For this review, take the finished solid that the model builds, in its own axes (mm). Face numbers are marked on the shaded views. A direction names the side the tool comes from. Coordinates: 2 decimals unless noted, no trailing zeros. Loops run counter-clockwise (first coordinate to the right, second up) from the corner with the lowest first, then second, coordinate; pieces in that order, holes last. Notation, with made-up numbers: (-9.75, 36) - (13.25, 36) arc R24 ccw to (13.25, 60) - close; hole circle Ø4 at (72, -11). An arc over 180 degrees is marked (long way). One line per item, written item: value. Start each with the question number.
1. Take a section at C-C, the plane z = 5.5. State the section outline as (x, y) points, and give its area (3 significant figures).
2. For the marked faces 5, 6 and 7, list the 3-axis set-ups (+Z, -Z, +X, -X, +Y, -Y) from which the entire face can be reached by the end or side of a thin tool; tool diameter is ignored.
3. The part is to be moulded in two halves that separate along X. For the marked faces 1, 2, 3 and 4, say which applies: released by +X, released by -X, zero draft, split by the parting line, or undercut.
4. Insertion check: pin 1 (7.5 mm diameter, centred on x = 22.01, y = 142.89, fed in from -Z); pin 2 (1.8 mm diameter, centred on x = 22.5, y = 144, fed in from +Z). Each pin has a flat end and moves straight along its axis. Give the tip position at first contact, or say it passes through.
5. Take a section at B-B, the plane x = 15. State the section outline as (y, z) points.
6. To check wall thickness, follow line 1 (X direction, y = 162.5, z = 3.75); line 2 (Z direction, x = 9, y = 157); line 3 (X direction, y = 158.5, z = 0.75). State the ranges of each line that lie inside material, in increasing order. Write a range as from..to.
Autodesk Inventor part; units mm, degrees
ref_plane "YZ Plane" through (0, 0, 0) normal (1, 0, 0) x (0, 1, 0)
ref_plane "XZ Plane" through (0, 0, 0) normal (0, 1, 0) x (-1, 0, 0)
ref_plane "XY Plane" through (0, 0, 0) normal (0, 0, 1) x (1, 0, 0)
ref_plane "Work Plane1" through (52.5141, 202.7033, 6.4479) normal (0, 0, -1) x (0, 1, 0)
sketch "Sketch1" plane through (52.5141, 202.7033, 6.4479) normal (0, 0, -1) x (0, 1, 0)
  circle A0 centre (-59.8114, -30.5) radius 1.4 construction
  circle A1 centre (-38.8114, -18.3756) radius 1.4
  circle A2 centre (-38.8114, -42.6244) radius 1.4 construction
  circle A3 centre (41, 0) radius 1.65
  circle A4 centre (-9, 0) radius 1.65
  circle A5 centre (-9, 50) radius 1.65
  circle A6 centre (41, 50) radius 1.65
  circle A7 centre (16, 50) radius 1.65
  circle A8 centre (-9, 25) radius 1.65
  circle A9 centre (16, 0) radius 1.65
  circle A10 centre (41, 25) radius 1.65
  line L0 (80, 55) -> (-80, 55)
  line L1 (-80, 55) -> (-80, -55)
  line L2 (-80, -55) -> (80, -55)
  line L3 (80, -55) -> (80, 55)
  line L4 (-36.5, 0) -> (-36.5, -50)
  line L5 (-14, 0) -> (-36.5, 0)
  line L6 (-14, -5) -> (-14, 0)
  line L7 (72, -5) -> (-14, -5)
  line L8 (72, -50) -> (72, -5)
  line L9 (-36.5, -50) -> (72, -50)
  line L10 (-4, 45) -> (-4, 5)
  line L11 (36, 45) -> (-4, 45)
  line L12 (36, 5) -> (36, 45)
  line L13 (-4, 5) -> (36, 5)
  line L14 (-64.5989, -17.0433) -> (-64.5989, -57.0433) construction
  line L15 (-64.5989, -57.0433) -> (-34.5989, -57.0433) construction
  line L16 (-34.5989, -57.0433) -> (-34.5989, -17.0433) construction
  line L17 (-34.5989, -17.0433) -> (-64.5989, -17.0433) construction
  line L18 (-34.8114, -13.0433) -> (-63.8114, -13.0433)
  line L19 (-63.8114, -13.0433) -> (-63.8114, -52.6244)
  line L20 (-63.8114, -52.6244) -> (-34.8114, -52.6244)
  line L21 (-34.8114, -52.6244) -> (-34.8114, -13.0433)
  circle A11 centre (-59.8114, -30.5) radius 2.95
  circle A12 centre (-38.8114, -18.3756) radius 2.95
  circle A13 centre (-38.8114, -42.6244) radius 2.95 construction
  line L22 (-36.5, -35.1157) -> (-41.75, -35.1157) construction
  line L23 (-41.75, -35.1157) -> (-41.75, -38.5657) construction
  line L24 (-41.75, -38.5657) -> (-56.86, -38.5657) construction
  line L25 (-56.86, -38.5657) -> (-56.86, -35.1157) construction
  line L26 (-56.86, -35.1157) -> (-60.26, -35.1157) construction
  line L27 (-60.26, -35.1157) -> (-60.26, -52.0657) construction
  line L28 (-60.26, -52.0657) -> (-36.5, -52.0657) construction
  line L29 (-36.5, -52.0657) -> (-36.5, -35.1157) construction
  line L30 (-41.75, -28.3657) -> (-36.5, -28.3657) construction
  line L31 (-36.5, -28.3657) -> (-36.5, -25.0657) construction
  line L32 (-36.5, -25.0657) -> (-60.26, -25.0657) construction
  line L33 (-60.26, -25.0657) -> (-60.26, -28.3657) construction
  line L34 (-60.26, -28.3657) -> (-56.86, -28.3657) construction
  line L35 (-56.86, -28.3657) -> (-56.86, -27.0942) construction
  line L36 (-56.86, -27.0942) -> (-41.75, -27.0942) construction
  line L37 (-41.75, -27.0942) -> (-41.75, -28.3657) construction
  line L38 (-56.86, -35.1157) -> (-60.26, -35.1157) construction
  line L39 (-56.86, -38.5657) -> (-56.86, -35.1157) construction
  line L40 (-41.75, -38.5657) -> (-56.86, -38.5657) construction
  line L41 (-41.75, -35.1157) -> (-41.75, -38.5657) construction
  line L42 (-36.5, -35.1157) -> (-41.75, -35.1157) construction
  line L43 (-36.5, -35.05) -> (-36.5, -35.1157) construction
  line L44 (-36.5, -35.05) -> (-56.86, -35.05) construction
  line L45 (-36.5, -34.78) -> (-36.5, -35.05) construction
  line L46 (-36.5, -34.78) -> (-56.86, -34.78) construction
  line L47 (-36.5, -34.51) -> (-36.5, -34.78) construction
  line L48 (-36.5, -34.51) -> (-56.86, -34.51) construction
  line L49 (-36.5, -34.24) -> (-36.5, -34.51) construction
  line L50 (-36.5, -34.24) -> (-56.86, -34.24) construction
  line L51 (-36.5, -33.97) -> (-36.5, -34.24) construction
  line L52 (-36.5, -33.97) -> (-56.86, -33.97) construction
  line L53 (-36.5, -33.7) -> (-36.5, -33.97) construction
  line L54 (-36.5, -33.7) -> (-56.86, -33.7) construction
  line L55 (-36.5, -33.43) -> (-36.5, -33.7) construction
  line L56 (-36.5, -33.43) -> (-56.86, -33.43) construction
  line L57 (-36.5, -33.16) -> (-36.5, -33.43) construction
  line L58 (-36.5, -33.16) -> (-56.86, -33.16) construction
  line L59 (-36.5, -32.89) -> (-36.5, -33.16) construction
  line L60 (-36.5, -32.89) -> (-56.86, -32.89) construction
  line L61 (-36.5, -32.62) -> (-36.5, -32.89) construction
  line L62 (-36.5, -32.62) -> (-56.86, -32.62) construction
  line L63 (-36.5, -32.35) -> (-36.5, -32.62) construction
  line L64 (-36.5, -32.35) -> (-56.86, -32.35) construction
  line L65 (-36.5, -32.08) -> (-36.5, -32.35) construction
  line L66 (-36.5, -32.08) -> (-56.86, -32.08) construction
  line L67 (-36.5, -31.81) -> (-36.5, -32.08) construction
  line L68 (-36.5, -31.81) -> (-56.86, -31.81) construction
  line L69 (-36.5, -31.54) -> (-36.5, -31.81) construction
  line L70 (-36.5, -31.54) -> (-56.86, -31.54) construction
  line L71 (-36.5, -31.27) -> (-36.5, -31.54) construction
  line L72 (-36.5, -31.27) -> (-56.86, -31.27) construction
  line L73 (-36.5, -31) -> (-36.5, -31.27) construction
  line L74 (-36.5, -31) -> (-56.86, -31) construction
  line L75 (-36.5, -30.73) -> (-36.5, -31) construction
  line L76 (-36.5, -30.73) -> (-56.86, -30.73) construction
  line L77 (-36.5, -30.46) -> (-36.5, -30.73) construction
  line L78 (-36.5, -30.46) -> (-56.86, -30.46) construction
  line L79 (-36.5, -30.19) -> (-36.5, -30.46) construction
  line L80 (-36.5, -30.19) -> (-56.86, -30.19) construction
  line L81 (-36.5, -29.92) -> (-36.5, -30.19) construction
  line L82 (-36.5, -29.92) -> (-56.86, -29.92) construction
  line L83 (-36.5, -29.65) -> (-36.5, -29.92) construction
  line L84 (-36.5, -29.65) -> (-56.86, -29.65) construction
  line L85 (-36.5, -29.38) -> (-36.5, -29.65) construction
  line L86 (-36.5, -29.38) -> (-56.86, -29.38) construction
  line L87 (-36.5, -29.11) -> (-36.5, -29.38) construction
  line L88 (-36.5, -29.11) -> (-56.86, -29.11) construction
  line L89 (-36.5, -28.84) -> (-36.5, -29.11) construction
  line L90 (-36.5, -28.84) -> (-56.86, -28.84) construction
  line L91 (-36.5, -28.3657) -> (-36.5, -28.84) construction
  line L92 (-41.75, -28.3657) -> (-36.5, -28.3657) construction
  line L93 (-41.75, -27.0942) -> (-41.75, -28.3657) construction
  line L94 (-56.86, -27.0942) -> (-41.75, -27.0942) construction
  line L95 (-56.86, -28.3657) -> (-56.86, -27.0942) construction
  line L96 (-60.26, -28.3657) -> (-56.86, -28.3657) construction
  line L97 (-60.26, -35.1157) -> (-60.26, -28.3657) construction
  line L98 (-60.26, -25.0657) -> (-36.5, -25.0657) construction
  line L99 (-36.5, -25.0657) -> (-36.5, -52.0657) construction
  line L100 (-60.26, -52.0657) -> (-60.26, -25.0657) construction
  line L101 (-57.1632, -22.5233) -> (-33.4032, -22.5233) construction
  line L102 (-33.4032, -22.5233) -> (-33.4032, -49.5233) construction
  line L103 (-33.4032, -49.5233) -> (-57.1632, -49.5233) construction
  line L104 (-57.1632, -49.5233) -> (-57.1632, -22.5233) construction
  circle A14 centre (-38.8114, -42.6244) radius 2.95
  point P0 (-202.7033, -52.5141)
  point P1 (-56.7146, -27.9576)
  dimension "d0" = 4
  dimension "d2" = 4
  dimension "d3" = 4
  dimension "d4" = 5.9
  dimension "d5" = 5.9
  dimension "d6" = 5.9
  dimension "d10" = 10
extrude "Extrusion1" add sketch "Sketch1" along normal blind 4 contours L18 L21 L9 L4 A14 A12 | L4 A12 A14 L9 L21 L20 L19 L18
sketch "Sketch2" plane through (52.5141, 202.7033, 2.4479) normal (0, 0, -1) x (-1, 0, 0)
  circle A0 centre (42.6244, -38.8114) radius 2.95
  circle A1 centre (18.3756, -38.8114) radius 2.95
  circle A2 centre (30.5, -59.8114) radius 2.95
  line L0 (13.0433, -34.8114) -> (13.0433, -63.8114)
  line L1 (13.0433, -63.8114) -> (52.6244, -63.8114)
  line L2 (52.6244, -63.8114) -> (52.6244, -34.8114)
  line L3 (52.6244, -34.8114) -> (13.0433, -34.8114)
  point P0 (52.5141, -202.7033)
extrude "Extrusion2" add sketch "Sketch2" along normal blind 1.5 contours A0 | A1 | A2 | L3 L2 L1 L0
sketch "Sketch3" plane through (-0.1103, 138.8919, 6.4479) normal (0, -1, 0) x (1, 0, 0)
  line L0 (39.581, 0) -> (0, 0)
  line L1 (0, 0) -> (0, -5.5)
  line L2 (39.581, -5.5) -> (0, -5.5)
  line L3 (39.581, 0) -> (39.581, -5.5)
  line L4 (17.5087, -7.4479) -> (17.5087, -6.8479) construction
  line L5 (17.5087, -6.8479) -> (24.2587, -6.8479) construction
  line L6 (24.2587, -6.8479) -> (24.2587, -7.4479) construction
  line L7 (27.5587, -7.4479) -> (24.2587, -7.4479) construction
  line L8 (27.5587, -6.4479) -> (27.5587, -7.4479) construction
  line L9 (27.5587, -6.4479) -> (0.5587, -6.4479) construction
  line L10 (0.5587, -6.4479) -> (0.5587, -7.4479) construction
  line L11 (17.5087, -7.4479) -> (0.5587, -7.4479) construction
  line L12 (39.581, 0) -> (39.581, -5.5)
  line L13 (39.581, -5.5) -> (34.8694, -5.5)
  line L14 (34.8694, -5.5) -> (34.8694, -6)
  line L15 (34.8694, -6.8) -> (39.581, -6.8)
  line L16 (39.581, -6.8) -> (39.581, -5.5)
  line L17 (39.581, -6.8) -> (32.6714, -6.8)
  line L18 (32.6714, -6.8) -> (34.8694, -6)
  line L19 (12.6726, -5.5) -> (12.6726, -6.5)
  line L20 (0, 0) -> (0, -5.5)
  line L21 (0, -5.5) -> (8.1109, -5.5)
  line L22 (8.1109, -6.8) -> (0, -6.8)
  line L23 (0, -6.8) -> (0, -5.5)
  line L24 (9.7957, -6.8) -> (8.1109, -6.8)
  line L25 (0, -5.5) -> (39.581, -5.5)
  line L26 (9.7957, -6.8) -> (7.5977, -6)
  line L27 (7.5977, -6) -> (7.5977, -5.5)
  line L28 (8.8957, -5.5) -> (33.4957, -5.5) construction
  line L29 (33.4957, -5.5) -> (33.4957, -6.5) construction
  line L30 (33.4957, -6.5) -> (8.8957, -6.5) construction
  line L31 (8.8957, -6.5) -> (8.8957, -5.5) construction
  point P0 (8.981, -5.5)
  dimension "d42" = 1.3
  dimension "d43" = 110
  dimension "d45" = 0.5
  dimension "d46" = 0.5
  dimension "d47" = 110
  dimension "d48" = 24.6
  dimension "d49" = 1
  dimension "d50" = 0.9
  dimension "d51" = 0
extrude "Extrusion3" add sketch "Sketch3" against normal up to surface (29 mm away) contours L16 L15 L17 L18 L14 L2 | L2 L27 L26 L24 L22 L23
sketch "Sketch6" plane through (52.5141, 202.7033, 6.4479) normal (0, 0, 1) x (1, 0, 0)
  line L0 (-13.0433, -34.8114) -> (-13.0433, -63.8114)
  line L1 (-52.6244, -34.8114) -> (-13.0433, -34.8114)
  line L2 (-52.6244, -63.8114) -> (-52.6244, -34.8114)
  line L3 (-13.0433, -63.8114) -> (-52.6244, -63.8114)
  line L4 (-23.5962, -45.8071) -> (-17.5454, -39.7563)
  line L5 (-17.5454, -39.7563) -> (-19.6668, -37.635)
  line L6 (-19.6668, -37.635) -> (-25.7175, -43.6858)
  line L7 (-25.7175, -43.6858) -> (-23.5962, -45.8071)
  line L8 (-23.5962, -45.8071) -> (-19.6668, -37.635) construction
  line L9 (-17.5454, -39.7563) -> (-25.7175, -43.6858) construction
  line L10 (-39.0797, -45.8071) -> (-43.9064, -40.9803)
  line L11 (-43.9064, -40.9803) -> (-41.7851, -38.859)
  line L12 (-41.7851, -38.859) -> (-36.9583, -43.6858)
  line L13 (-36.9583, -43.6858) -> (-39.0797, -45.8071)
  line L14 (-39.0797, -45.8071) -> (-41.7851, -38.859) construction
  line L15 (-43.9064, -40.9803) -> (-36.9583, -43.6858) construction
  line L16 (-25.7175, -43.6858) -> (-36.9583, -43.6858)
  line L17 (-23.5962, -45.8071) -> (-23.5962, -49.9899)
  line L18 (-23.5962, -49.9899) -> (-39.0797, -49.9899)
  line L19 (-39.0797, -49.9899) -> (-39.0797, -45.8071)
  point P0 (-52.5141, -202.7033)
  point P1 (-21.6315, -41.7211)
  point P2 (-40.4324, -42.333)
  dimension "d35" = 3
  dimension "d36" = 3
  dimension "d37" = 45
  dimension "d38" = 0
extrude "Extrusion6" cut sketch "Sketch6" against normal up to surface (4 mm away) contours L7 L6 L5 L4 | L17 L18 L19 L13 L16 L7 | L13 L10 L11 L12
properties part number "cellSTORM_v5_chiptray_new_0_22.4"
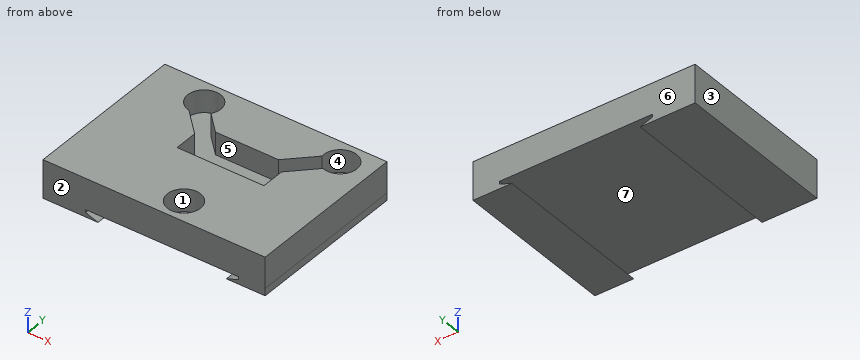
Solutions:
1. outline: (-0.11, 138.89) - (39.47, 138.89) - (39.47, 167.89) - (-0.11, 167.89) - close; hole (9.34, 160.99) - (13.43, 156.9) - (13.43, 152.71) - (28.92, 152.71) - (28.92, 156.9) - (33.14, 161.12) arc R2.95 ccw (long way) to (31.22, 163.44) - (26.8, 159.02) - (15.56, 159.02) - (12.33, 162.24) arc R2.95 ccw (long way) to start; hole circle Ø5.9 at (22.01, 142.89)
1. area: 941 mm2
2. face 5: +Z
2. face 6: +Z, -Z, +X, -X, +Y
2. face 7: +Y, -Y
3. face 1: undercut
3. face 2: zero draft
3. face 3: released by -X
3. face 4: undercut
4. pin 1: z = 0.95
4. pin 2: z = 2.45
5. outline: (138.89, 0.95) - (167.89, 0.95) - (167.89, 6.45) - (159.57, 6.45) - (159.57, 2.45) - (152.71, 2.45) - (152.71, 6.45) - (138.89, 6.45) - close
6. line 1: -0.11..7.29, 12.49..30.28, 36.74..39.47
6. line 2: -0.35..-0.1, 0.95..6.45
6. line 3: -0.11..7.49, 34.76..39.47
